```python
from build123d import *

# Parameters (mm, degrees)
F0_R     = 12.825
F1_DEPTH = 5


with BuildPart() as f1:
    # F0 (on Front) → F1 (new body)
    with BuildSketch(Plane.XZ):
        with BuildLine():
            ThreePointArc((-1.513547, -4.804002), (0, -0.145783), (1.513547, -4.804002))
            Line((1.513547, -4.804002), (2.98301, -6.826544))
            ThreePointArc((2.98301, -6.826544), (4.402496, -5.245392), (5.050221, -3.221673))
            ThreePointArc((5.050221, -3.221673), (6.891336, 3.645865), (10.835703, 9.561502))
            ThreePointArc((10.835703, 9.561502), (0, 34.504217), (-10.835703, 9.561502))
            ThreePointArc((-10.835703, 9.561502), (-6.891336, 3.645865), (-5.050221, -3.221673))
            ThreePointArc((-5.050221, -3.221673), (-4.402496, -5.245392), (-2.98301, -6.826544))
            Line((-2.98301, -6.826544), (-1.513547, -4.804002))
        make_face()
        with Locations((0, 19.679217)):
            Circle(F0_R, mode=Mode.SUBTRACT)
    extrude(amount=F1_DEPTH)


solid = f1.part
```
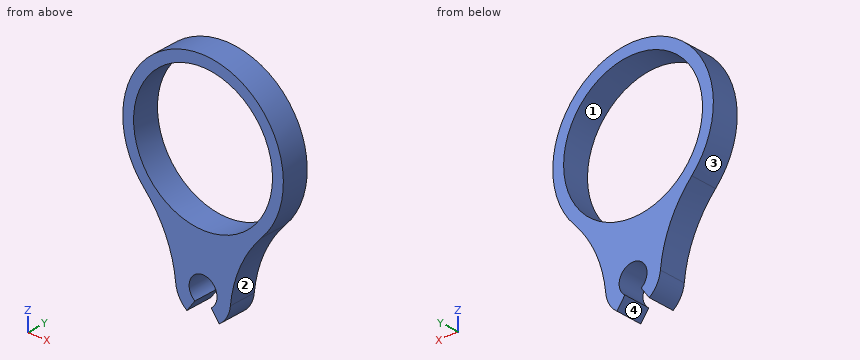
The model under review builds one solid part; all positions refer to its coordinate system, in mm. Face numbers are marked on the shaded views. Coordinates: 2 decimals unless noted, no trailing zeros. Order: outer loops, then holes, each group sorted by start corner. A loop starts at its lowest first (then second) coordinate and runs counter-clockwise, first axis right, second up. Notation, with made-up numbers: (39.25, -8.75) -> (96.25, -8.75) arc R11 ccw to (96.25, 8.25) -> close; hole circle Ø5 at (84.25, 10.25). An arc over 180 degrees is marked (long way). Answer in a Markdown table with one row per item. Add a question column.
Item 1: Clearance check with flat-ended pins moving along their axes: pin 1 (2 mm diameter, centred on y = -2.5, z = 2.5, fed in from -X); pin 2 (3 mm diameter, centred on y = -2.5, z = 28.5, fed in from -X); pin 3 (2 mm diameter, centred on x = 6.5, y = -3, fed in from +Z). State where each tip first meets the part, or that it passes through.
Item 2: We need section D-D on z = 2. Write out the cut boundary in (x, y).
Item 3: Mouldability with a two-part tool opening along X and no side actions: class the marked faces 1, 2, 3 and 4 as +X half, -X half, draft (parallel to the pull), parting line (faces both ways), or undercut.
Item 4: We need section B-B on z = 22.5. Write out the cut boundary in (x, y), plus the area to 3 significant figures.
Item 5: We need section A-A on x = 0. Write out the cut boundary in (y, z).
Item 6: To check wall thickness, follow probe 1 along Z at (x, y) = (0, -3.6); probe 2 along X at (y, z) = (-1.3, 20); probe 3 along Z at (x, y) = (-10, -4.45). State the ranges of each line that lie inside material, in increasing order.
Final values:
| question | item | result |
|---|---|---|
| 1 | pin 1 | stops at x = -6.83 |
| 1 | pin 2 | stops at x = -12.89 |
| 1 | pin 3 | stops at z = 33.45 |
| 2 | outline | (-6.23, -5) -> (6.23, -5) -> (6.23, 0) -> (-6.23, 0) -> close |
| 3 | face 1 | undercut |
| 3 | face 2 | +X half |
| 3 | face 3 | parting line |
| 3 | face 4 | undercut |
| 4 | outline | (-14.55, -5) -> (-12.51, -5) -> (-12.51, 0) -> (-14.55, 0) -> close; (12.51, -5) -> (14.55, -5) -> (14.55, 0) -> (12.51, 0) -> close |
| 4 | area | 20.4 mm2 |
| 5 | outline | (-5, -0.15) -> (0, -0.15) -> (0, 6.85) -> (-5, 6.85) -> close; (-5, 32.5) -> (0, 32.5) -> (0, 34.5) -> (-5, 34.5) -> close |
| 6 | probe 1 | z = -0.15 to 6.85, 32.5 to 34.5 |
| 6 | probe 2 | x = -14.82 to -12.82, 12.82 to 14.82 |
| 6 | probe 3 | z = 8.61 to 11.65, 27.71 to 30.62 |
